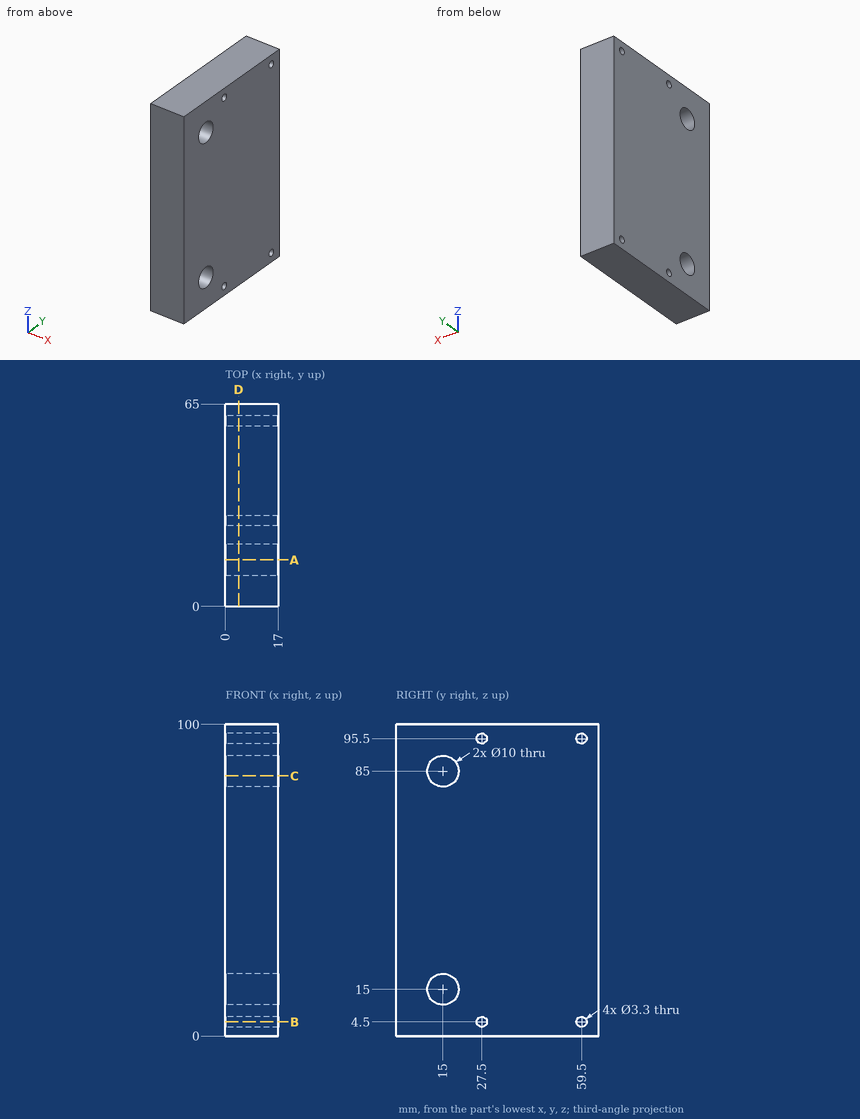
Part print with two shaded views. Sizes in mm from the minimum x, y, z corner. Round coordinates to 2 decimals unless told otherwise and drop trailing zeros. Loops run counter-clockwise (first coordinate to the right, second up) from the corner with the lowest first, then second, coordinate; pieces in that order, holes last.
Item 1: Saw through at C-C (z = 83.5). List the corners of the cut face in (x, y), then the cut area to 3 significant figures.
Item 2: Saw through at B-B (z = 4.5). List the corners of the cut face in (x, y), then the cut area to 3 significant figures.
Item 3: Saw through at D-D (x = 4.25). List the corners of the cut face in (y, z).
Item 4: Saw through at A-A (y = 15). List the corners of the cut face in (x, z), then the cut area to 3 significant figures.
Item 5: Drill centre lines: line 1 along Z through (x, y) = (13, 27.5); line 2 along Z through (x, y) = (7.75, 15); line 3 along Y through (x, z) = (1.5, 13.5). Where is each one in solid material? Low to high.
Item 6: Pin check, flat tips, straight feed: P1, Ø8, axis at y = 15, z = 15, coming from the -X side; P2, Ø11.5, axis at y = 15, z = 85, coming from the -X side. Stop position of each tip, or through.
Worked answers:
1. outline: (0, 0) - (17, 0) - (17, 10.23) - (0, 10.23) - close; (0, 19.77) - (17, 19.77) - (17, 65) - (0, 65) - close
1. area: 943 mm2
2. outline: (0, 0) - (17, 0) - (17, 25.85) - (0, 25.85) - close; (0, 29.15) - (17, 29.15) - (17, 57.85) - (0, 57.85) - close; (0, 61.15) - (17, 61.15) - (17, 65) - (0, 65) - close
2. area: 993 mm2
3. outline: (0, 0) - (65, 0) - (65, 100) - (0, 100) - close; hole circle Ø10 at (15, 15); hole circle Ø10 at (15, 85); hole circle Ø3.3 at (27.5, 4.5); hole circle Ø3.3 at (27.5, 95.5); hole circle Ø3.3 at (59.5, 4.5); hole circle Ø3.3 at (59.5, 95.5)
4. outline: (0, 0) - (17, 0) - (17, 10) - (0, 10) - close; (0, 20) - (17, 20) - (17, 80) - (0, 80) - close; (0, 90) - (17, 90) - (17, 100) - (0, 100) - close
4. area: 1,360 mm2
5. line 1: z = 0 to 2.85, 6.15 to 93.85, 97.15 to 100
5. line 2: z = 0 to 10, 20 to 80, 90 to 100
5. line 3: y = 0 to 10.23, 19.77 to 65
6. P1: passes through
6. P2: stops at x = 0
